Check sheet for the modelled part. Datum: model origin and axes. Units: mm. Give positions to 0.01 mm unless a question says otherwise; leave off trailing zeros. Write each loop counter-clockwise with the first axis right and the second up, starting at its lowest first coordinate (ties: lowest second). Pieces come first, ordered by that corner, then holes. Notation, with made-up numbers: M -37,-7 L -26,-7 A17 ccw -26,6 Z; hole C 27.5,-29 d11. An arc over 180 degrees is marked long. Write item = value, one per line. Start each with the question number.
1) Sectioned sample at C-C, the plane x = -50. Record the cut outline in (y, z), then the cut area to 3 significant figures.
2) Sectioned sample at B-B, the plane y = -54. Record the cut outline in (x, z).
3) Sectioned sample at D-D, the plane z = 2.45. Count the separate pieces of the cut face and the enclosed holes in it, then the cut area to 3 significant figures.
4) Gauge pin test, flat end, axial feed: pin 1 (1 mm diameter, centred on x = -53.5, y = -41.5, fed in from -Z). Record the tip position at first contact, or that the pin passes through.
5) Scan lines: L1, parallel to Y at x = 55.5, z = 0.7; L2, parallel to X at y = 15.5, z = 0.7; L3, parallel to X at y = -72.5, z = 1.55. Record each from-to range of solid material in increasing order.
6) Sectioned sample at A-A, the plane x = 53. Record the cut outline in (y, z), then the cut area to 3 significant figures.
from build123d import *

# Parameters (mm, degrees)
SKETCH1_W           = 160
SKETCH1_H           = 142
SKETCH1_W_2         = 130
SKETCH1_H_2         = 3
SKETCH1_W_3         = 3
SKETCH1_H_3         = 128
SKETCH1_W_4         = 12
SKETCH1_H_4         = 19
BOSS_EXTRUDE1_DEPTH = 3


with BuildPart() as part:
    # Sketch1 → Boss-Extrude1 (new body)
    with BuildSketch(Plane.XY):
        with Locations((-2.653971439, -21.497313052)):
            Rectangle(SKETCH1_W, SKETCH1_H)
        with Locations((-2.653971439, -88.997313052)):
            Rectangle(SKETCH1_W_2, SKETCH1_H_2, mode=Mode.SUBTRACT)
        with Locations((-2.653971439, 46.002686948)):
            Rectangle(SKETCH1_W_2, SKETCH1_H_2, mode=Mode.SUBTRACT)
        with Locations((-79.153971439, -21.497313052)):
            Rectangle(SKETCH1_W_3, SKETCH1_H_3, mode=Mode.SUBTRACT)
        with Locations((73.846028561, -20.307455235)):
            Rectangle(SKETCH1_W_3, SKETCH1_H_3, mode=Mode.SUBTRACT)
        with Locations((43.346028561, -61.997313052)):
            Rectangle(SKETCH1_W_4, SKETCH1_H_2, mode=Mode.SUBTRACT)
        with Locations((43.346028561, -83.997313052)):
            Rectangle(SKETCH1_W_4, SKETCH1_H_2, mode=Mode.SUBTRACT)
        with Locations((43.346028561, 41.002686948)):
            Rectangle(SKETCH1_W_4, SKETCH1_H_2, mode=Mode.SUBTRACT)
        with Locations((8.846028561, -72.997313052)):
            Rectangle(SKETCH1_W_3, SKETCH1_H_4, mode=Mode.SUBTRACT)
        with Locations((43.346028561, 19.002686948)):
            Rectangle(SKETCH1_W_4, SKETCH1_H_2, mode=Mode.SUBTRACT)
        with Locations((8.846028561, 30.002686948)):
            Rectangle(SKETCH1_W_3, SKETCH1_H_4, mode=Mode.SUBTRACT)
        with Locations((-14.153971439, -72.997313052)):
            Rectangle(SKETCH1_W_3, SKETCH1_H_4, mode=Mode.SUBTRACT)
        with Locations((-48.653971439, -83.997313052)):
            Rectangle(SKETCH1_W_4, SKETCH1_H_2, mode=Mode.SUBTRACT)
        with Locations((-48.653971439, -61.997313052)):
            Rectangle(SKETCH1_W_4, SKETCH1_H_2, mode=Mode.SUBTRACT)
        with Locations((-48.653971439, 19.002686948)):
            Rectangle(SKETCH1_W_4, SKETCH1_H_2, mode=Mode.SUBTRACT)
        with Locations((-48.653971439, 41.002686948)):
            Rectangle(SKETCH1_W_4, SKETCH1_H_2, mode=Mode.SUBTRACT)
        with Locations((-14.153971439, 30.002686948)):
            Rectangle(SKETCH1_W_3, SKETCH1_H_4, mode=Mode.SUBTRACT)
    extrude(amount=BOSS_EXTRUDE1_DEPTH)


solid = part.part
Data:
q1.outline = M -92.5,0 L -90.5,0 L -90.5,3 L -92.5,3 Z; M -87.5,0 L -85.5,0 L -85.5,3 L -87.5,3 Z; M -82.5,0 L -63.5,0 L -63.5,3 L -82.5,3 Z; M -60.5,0 L 17.5,0 L 17.5,3 L -60.5,3 Z; M 20.5,0 L 39.5,0 L 39.5,3 L 20.5,3 Z; M 42.5,0 L 44.5,0 L 44.5,3 L 42.5,3 Z; M 47.5,0 L 49.5,0 L 49.5,3 L 47.5,3 Z
q1.area = 372 mm2
q2.outline = M -82.65,0 L -80.65,0 L -80.65,3 L -82.65,3 Z; M -77.65,0 L 72.35,0 L 72.35,3 L -77.65,3 Z; M 75.35,0 L 77.35,0 L 77.35,3 L 75.35,3 Z
q3.separate_pieces = 1
q3.enclosed_holes = 16
q3.area = 20,700 mm2
q4.pin_1 = 0
q5.L1 = -92.5 to -90.5, -87.5 to 44.5, 47.5 to 49.5
q5.L2 = -82.65 to -80.65, -77.65 to 72.35, 75.35 to 77.35
q5.L3 = -82.65 to -80.65, -77.65 to -15.65, -12.65 to 7.35, 10.35 to 72.35, 75.35 to 77.35
q6.outline = M -92.5,0 L -90.5,0 L -90.5,3 L -92.5,3 Z; M -87.5,0 L 44.5,0 L 44.5,3 L -87.5,3 Z; M 47.5,0 L 49.5,0 L 49.5,3 L 47.5,3 Z
q6.area = 408 mm2
